Design review of the part built by this model. Coordinates are the model's own, in mm. Give positions to 0.01 mm unless a question says otherwise; leave off trailing zeros. Write each loop counter-clockwise with the first axis right and the second up, starting at its lowest first coordinate (ties: lowest second). Pieces come first, ordered by that corner, then holes. Notation, with made-up numbers: (-38.5, 6) -> (12.5, 6) arc R18 ccw to (12.5, 41) -> close; hole circle Ø8 at (50, -28). An arc over 180 degrees is marked (long way). Put each result on its own line as item: value. Start each with the question number.
from build123d import *

# Parameters (mm, degrees)
BOSS_EXTRUDE1_DEPTH = 6
FILLET1_R           = 0.5
SKETCH4_R           = 6
BOSS_EXTRUDE2_DEPTH = 6
SKETCH3_R           = 2
SKETCH3_R_2         = 6
CUT_EXTRUDE1_DEPTH  = 284.694910827
CUT_EXTRUDE2_REACH  = 285.695
SKETCH6_R           = 1.55


with BuildPart() as part:
    # Sketch2 → Boss-Extrude1 (new body)
    with BuildSketch(Plane(origin=(0, 0, 0), x_dir=(0, 0, -1), z_dir=(1, 0, 0))):
        Polygon((-30.67492643, 30.67492643), (-30.67492643, 257.67492643), (-5.67492643, 282.67492643), (-5.67492643, 5.67492643), align=None)
    extrude(amount=BOSS_EXTRUDE1_DEPTH)

    # Fillet1
    fillet1_edges = [part.edges().sort_by_distance(p)[0] for p in [
        (3, 282.67492643, 5.67492643),
        (3, 5.67492643, 5.67492643),
    ]]
    fillet(fillet1_edges, radius=FILLET1_R)

    # Sketch4 → Boss-Extrude2 (add)
    with BuildSketch(Plane(origin=(6, 0, 0), x_dir=(0, 0, -1), z_dir=(1, 0, 0))):
        with Locations((-17.67492643, 270.67492643)):
            Circle(SKETCH4_R)
    extrude(amount=-BOSS_EXTRUDE2_DEPTH)

    # Sketch3 → Cut-Extrude1 (cut, through all)
    with BuildSketch(Plane(origin=(6, 0, 0), x_dir=(0, 0, -1), z_dir=(1, 0, 0))):
        with Locations((-17.67492643, 270.67492643)):
            Circle(SKETCH3_R)
        with Locations((-17.67492643, 17.67492643)):
            Circle(SKETCH3_R_2)
    extrude(amount=-CUT_EXTRUDE1_DEPTH, mode=Mode.SUBTRACT)

    # Sketch6 → Cut-Extrude2 (cut, up to next)
    with BuildSketch(Plane(origin=(6, 0, 0), x_dir=(0, 0, -1), z_dir=(1, 0, 0)), mode=Mode.PRIVATE) as cut_extrude2_sk1:
        with Locations((-18.17492643, 244.17492643)):
            Circle(SKETCH6_R)
    cut_extrude2_tool1 = extrude(cut_extrude2_sk1.sketch, amount=-CUT_EXTRUDE2_REACH, mode=Mode.PRIVATE) & part.part
    # Sketch6 → Cut-Extrude2 (cut, up to next)
    with BuildSketch(Plane(origin=(6, 0, 0), x_dir=(0, 0, -1), z_dir=(1, 0, 0)), mode=Mode.PRIVATE) as cut_extrude2_sk2:
        with Locations((-18.17492643, 224.17492643)):
            Circle(SKETCH6_R)
    cut_extrude2_tool2 = extrude(cut_extrude2_sk2.sketch, amount=-CUT_EXTRUDE2_REACH, mode=Mode.PRIVATE) & part.part
    # Sketch6 → Cut-Extrude2 (cut, up to next)
    with BuildSketch(Plane(origin=(6, 0, 0), x_dir=(0, 0, -1), z_dir=(1, 0, 0)), mode=Mode.PRIVATE) as cut_extrude2_sk3:
        with Locations((-18.17492643, 64.17492643)):
            Circle(SKETCH6_R)
    cut_extrude2_tool3 = extrude(cut_extrude2_sk3.sketch, amount=-CUT_EXTRUDE2_REACH, mode=Mode.PRIVATE) & part.part
    # Sketch6 → Cut-Extrude2 (cut, up to next)
    with BuildSketch(Plane(origin=(6, 0, 0), x_dir=(0, 0, -1), z_dir=(1, 0, 0)), mode=Mode.PRIVATE) as cut_extrude2_sk4:
        with Locations((-18.17492643, 44.17492643)):
            Circle(SKETCH6_R)
    cut_extrude2_tool4 = extrude(cut_extrude2_sk4.sketch, amount=-CUT_EXTRUDE2_REACH, mode=Mode.PRIVATE) & part.part
    add(cut_extrude2_tool1.solids().sort_by_distance((6, 244.174926, 18.174926))[0], mode=Mode.SUBTRACT)
    add(cut_extrude2_tool2.solids().sort_by_distance((6, 224.174926, 18.174926))[0], mode=Mode.SUBTRACT)
    add(cut_extrude2_tool3.solids().sort_by_distance((6, 64.174926, 18.174926))[0], mode=Mode.SUBTRACT)
    add(cut_extrude2_tool4.solids().sort_by_distance((6, 44.174926, 18.174926))[0], mode=Mode.SUBTRACT)


solid = part.part
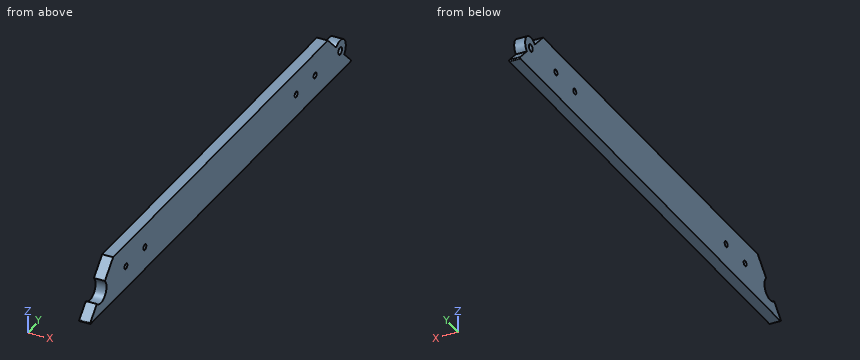
Q1. For pin 1 (3 mm diameter, centred on x = 2, z = 19, fed in from +Y); pin 2 (3 mm diameter, centred on x = 1, z = 16, fed in from -Y), all flat-tipped, find the tip position at first contact; note any pin that passes through.
Q2. Take a section at A-A on x = 2.75. Give the boundary of the cut face in (y, z), then the cut area to 3 significant figures.
Q3. Take a section at B-B on z = 26.25. Give the boundary of the cut face in (x, y), then the cut area to 3 significant figures.
Q4. To check wall thickness, follow probe 1 along Z at (x, y) = (0.55, 45); probe 2 along Y at (x, z) = (0.45, 22.5); probe 3 along Z at (x, y) = (1.6, 27). State the ranges of each line that lie inside material, in increasing order. Write a range as from..to.
Result:
1. pin 1: stops at y = 276.67
1. pin 2: stops at y = 22.77
2. outline: (6.53, 6.53) arc R0.5 ccw to (6.88, 5.67) -> (281.47, 5.67) arc R0.5 ccw to (281.82, 6.53) -> (274.92, 13.43) arc R6 ccw to (266.43, 21.92) -> (257.67, 30.67) -> (30.67, 30.67) -> (21.92, 21.92) arc R6 cw to (13.43, 13.43) -> close; hole circle Ø3.1 at (44.17, 18.17); hole circle Ø3.1 at (64.17, 18.17); hole circle Ø3.1 at (224.17, 18.17); hole circle Ø3.1 at (244.17, 18.17); hole circle Ø4 at (270.67, 17.67)
2. area: 6,260 mm^2
3. outline: (0, 26.25) -> (6, 26.25) -> (6, 262.1) -> (0, 262.1) -> close
3. area: 1,420 mm^2
4. probe 1: z = 5.67..16.86, 19.49..30.67
4. probe 2: y = 22.5..265.85, 267.11..274.24
4. probe 3: z = 5.67..27
